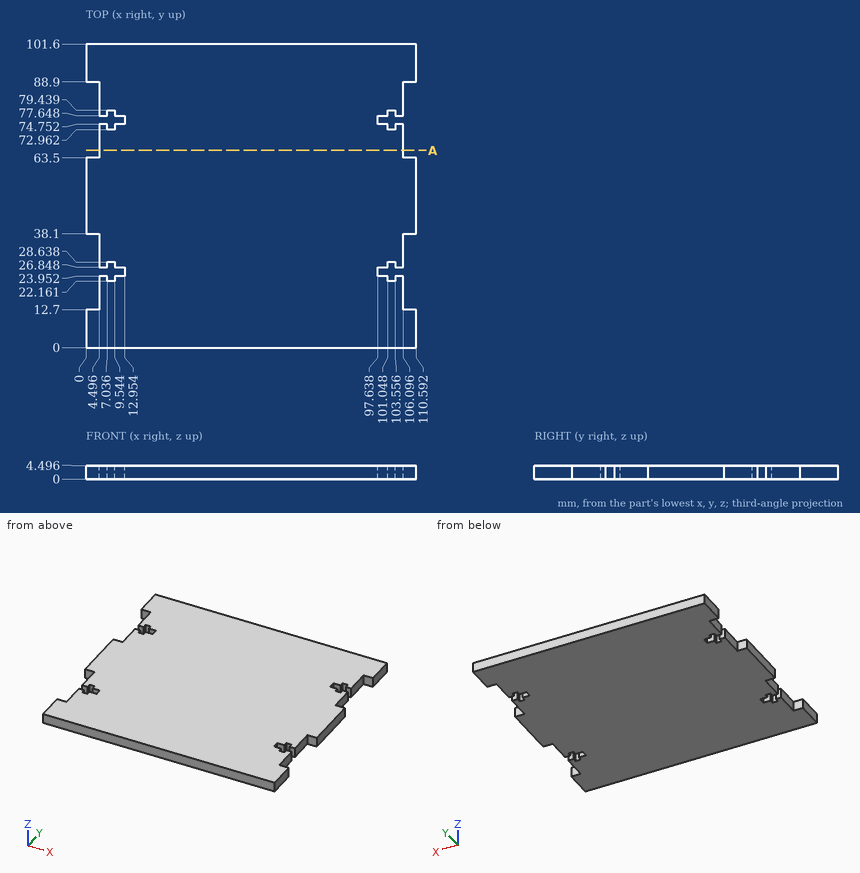
Could you check a few things on this drawing? It's one solid part, dimensions in mm from its lowest x, y, z. Coordinates: 2 decimals unless noted, no trailing zeros. Write each loop counter-clockwise with the first axis right and the second up, starting at its lowest first coordinate (ties: lowest second). Pieces come first, ordered by that corner, then holes.
Q1. Imagine slicing it at A-A, the plane y = 66. List the corners of the cut face in (x, z) for me (1 decimal).
Results found:
outline: (4.5, 0) - (106.1, 0) - (106.1, 4.5) - (4.5, 4.5) - close
Q2. For P1, Ø2, axis at y = 28, z = 2.5, coming from the -X side; P2, Ø0.9, axis at y = 28, z = 2, coming from the +X side, each with a flat end and sliding along its axis, tell me the tip position at first contact or that it passes through.
Results found:
P1: stops at x = 4.5
P2: stops at x = 106.1
Q3. Please list where these lines run through material, in increasing order: L1, parallel to X at y = 73.5, z = 4.2 (1 decimal); L2, parallel to Y at x = 11, z = 3.4; L3, parallel to X at y = 24.5, z = 1.65 (1 decimal).
Results found:
L1: x = 4.5 to 7, 9.5 to 101, 103.6 to 106.1
L2: y = 0 to 23.95, 26.85 to 74.75, 77.65 to 101.6
L3: x = 13 to 97.6
